Input: part model. Units: mm. Frame: model coordinates. A direction names the side the tool comes from. Coordinates: 2 decimals unless noted, no trailing zeros. Loops run counter-clockwise (first coordinate to the right, second up) from the corner with the lowest first, then second, coordinate; pieces in that order, holes last.
```python
from build123d import *

# Parameters (mm, degrees)
BOSS_EXTRUDE1_DEPTH     = 15
SKETCH2_R               = 10
BOSS_EXTRUDE2_DEPTH     = 9
CUT_EXTRUDE1_START      = -15
SKETCH3_R               = 3
CUT_EXTRUDE1_DEPTH      = 15
SKETCH4_W               = 41
SKETCH4_H               = 21
CUT_EXTRUDE2_DEPTH      = 9.6
SKETCH5_W               = 25
SKETCH5_H               = 4
CUT_EXTRUDE3_DEPTH      = 25
CUT_EXTRUDE4_DEPTH      = 127.840450961
CUT_EXTRUDE4_DEPTH_BACK = 127.840450961
SKETCH6_R               = 6
SKETCH7_R               = 3
CUT_EXTRUDE5_DEPTH      = 127.840450961
SKETCH8_R               = 1.325011821
CUT_EXTRUDE6_DEPTH      = 126.449192903


with BuildPart() as part:
    # Sketch1 → Boss-Extrude1 (new body)
    with BuildSketch(Plane(origin=(0, 0, 0), x_dir=(1, 0, 0), z_dir=(0, 1, 0))):
        with BuildLine():
            Line((0, 22.5), (100, 22.5))
            ThreePointArc((100, 22.5), (122.5, 0), (100, -22.5))
            Line((100, -22.5), (0, -22.5))
            ThreePointArc((0, -22.5), (-22.5, 0), (0, 22.5))
        make_face()
    extrude(amount=BOSS_EXTRUDE1_DEPTH)

    # Sketch2 → Boss-Extrude2 (add)
    with BuildSketch(Plane.XZ):
        with Locations(Location((0, 0, 0), (0, 0, 90))):
            Circle(SKETCH2_R)
    extrude(amount=BOSS_EXTRUDE2_DEPTH)

    # Sketch3 → Cut-Extrude1 (cut)
    with BuildSketch(Plane(origin=(0, 15, 0), x_dir=(1, 0, 0), z_dir=(0, 1, 0)).offset(CUT_EXTRUDE1_START)):
        with Locations(Location((0, 0, 0), (0, 0, 270))):
            Circle(SKETCH3_R)
    extrude(amount=CUT_EXTRUDE1_DEPTH, mode=Mode.SUBTRACT)

    # Sketch4 → Cut-Extrude2 (cut)
    with BuildSketch(Plane(origin=(0, 15, 0), x_dir=(1, 0, 0), z_dir=(0, 1, 0))):
        with Locations((10, 0)):
            Rectangle(SKETCH4_W, SKETCH4_H)
    extrude(amount=-CUT_EXTRUDE2_DEPTH, mode=Mode.SUBTRACT)

    # Sketch5 → Cut-Extrude3 (cut)
    with BuildSketch(Plane(origin=(-22.5, 15, 0), x_dir=(0, 0, 1), z_dir=(-1, 0, 0))):
        with Locations((0, -13)):
            Rectangle(SKETCH5_W, SKETCH5_H)
    extrude(amount=-CUT_EXTRUDE3_DEPTH, mode=Mode.SUBTRACT)

    # Sketch6 → Cut-Extrude4 (cut, two sides: drawn at the far end of the back side and taken through both)
    with BuildSketch(Plane(origin=(0, 15, 0), x_dir=(1, 0, 0), z_dir=(0, 1, 0)).offset(-CUT_EXTRUDE4_DEPTH_BACK)):
        with Locations(Location((100, 0, 0), (0, 0, 270))):
            Circle(SKETCH6_R)
    extrude(amount=CUT_EXTRUDE4_DEPTH + CUT_EXTRUDE4_DEPTH_BACK, mode=Mode.SUBTRACT)

    # Sketch7 → Cut-Extrude5 (cut, through all)
    with BuildSketch(Plane(origin=(0, 15, 0), x_dir=(1, 0, 0), z_dir=(0, 1, 0))):
        with Locations(Location((63.480653876, -6.00928668, 0), (0, 0, 270))):
            Circle(SKETCH7_R)
    extrude(amount=-CUT_EXTRUDE5_DEPTH, mode=Mode.SUBTRACT)

    # Sketch8 → Cut-Extrude6 (cut, through all)
    with BuildSketch(Plane.XZ):
        with Locations(Location((46.139135996, -8.030751211, 0), (0, 0, 270))):
            Circle(SKETCH8_R)
        with Locations(Location((46.323389896, 7.468153605, 0), (0, 0, 270))):
            Circle(SKETCH8_R)
        with Locations(Location((59.837962148, 15.058037455, 0), (0, 0, 270))):
            Circle(SKETCH8_R)
        with Locations(Location((73.168280499, 7.149016489, 0), (0, 0, 270))):
            Circle(SKETCH8_R)
        with Locations(Location((72.984026599, -8.349888327, 0), (0, 0, 270))):
            Circle(SKETCH8_R)
        with Locations(Location((59.469454347, -15.939772177, 0), (0, 0, 270))):
            Circle(SKETCH8_R)
    extrude(amount=-CUT_EXTRUDE6_DEPTH, mode=Mode.SUBTRACT)


solid = part.part
```
Item 1: Contact query for flat-ended pins moving along their axis: P1, Ø3, axis at y = -0.5, z = 7, coming from the -X side; P2, Ø22.5, axis at x = 60, z = -5, coming from the -Y side; P3, Ø3, axis at x = -12, y = 1, coming from the +Z side; P4, Ø7, axis at x = 63.48, z = 6.01, coming from the +Y side. Output: stop coordinate, or through.
Result:
P1: stops at x = -8.35
P2: stops at y = 0
P3: stops at z = 19.9
P4: stops at y = 15
Item 2: Mould query, pull axis X, two halves, no side actions, for faces 6 (the face through (2.5, 2, 7)), 7 (the face through (-8, 2, -12.5)), 8 (the face through (10, 10, -10.5)), 9 (the face through (66.455, 7.605, 5.619)). Classes: +X half, -X half, draft (parallel to the pull), parting line (faces both ways), or undercut.
Result:
face 6: -X half
face 7: draft
face 8: undercut
face 9: undercut
Item 3: Section query A-A (z = 0). Output: boundary loops of the cut face in (x, y).
Result:
outline: (-22.5, 4) - (-3, 4) - (-3, 5.4) - (-10.5, 5.4) - (-10.5, 15) - (-22.5, 15) - close; (-10, -9) - (10, -9) - (10, 0) - (94, 0) - (94, 15) - (30.5, 15) - (30.5, 5.4) - (3, 5.4) - (3, 0) - (-10, 0) - close; (106, 0) - (122.5, 0) - (122.5, 15) - (106, 15) - close
Item 4: Section query C-C (x = 12). Output: boundary loops of the cut face in (y, z), then the cut area to 3 significant figures.
Result:
outline: (0, -22.5) - (15, -22.5) - (15, -10.5) - (5.4, -10.5) - (5.4, 10.5) - (15, 10.5) - (15, 22.5) - (0, 22.5) - close
area: 473 mm2
Item 5: Section query B-B (y = 2.5). Count the separate pieces of the cut face and the enclosed holes in it, then the cut area to 3 significant figures.
Result:
separate pieces: 1
enclosed holes: 8
area: 5,320 mm2
Item 6: Reachability of faces 1 (the face through (74.482, 7.395, 7.322)), 2 (the face through (9.76, -4.44, -2.17)), 3 (the face through (3, 4, 0)), 4 (the face through (2.5, 2, -7)), 5 (the face through (49, 7, -22.5)) from +Z, -Z, +X, -X, +Y, -Y: full face, straight path, thin tool, end or side. Return the list, or none.
Result:
face 1: +Y, -Y
face 2: -Y
face 3: +Y
face 4: -X
face 5: -Z, +X, -X, +Y, -Y
Item 7: Line query: L1, parallel to X at y = 8, z = 0; L2, parallel to X at y = 1, z = 0; L3, parallel to Z at x = 0, y = 12.75. Output: solid intervals per line, ascending.
Result:
L1: x = -22.5 to -10.5, 30.5 to 94, 106 to 122.5
L2: x = 3 to 94, 106 to 122.5
L3: z = -22.5 to -10.5, 10.5 to 22.5
